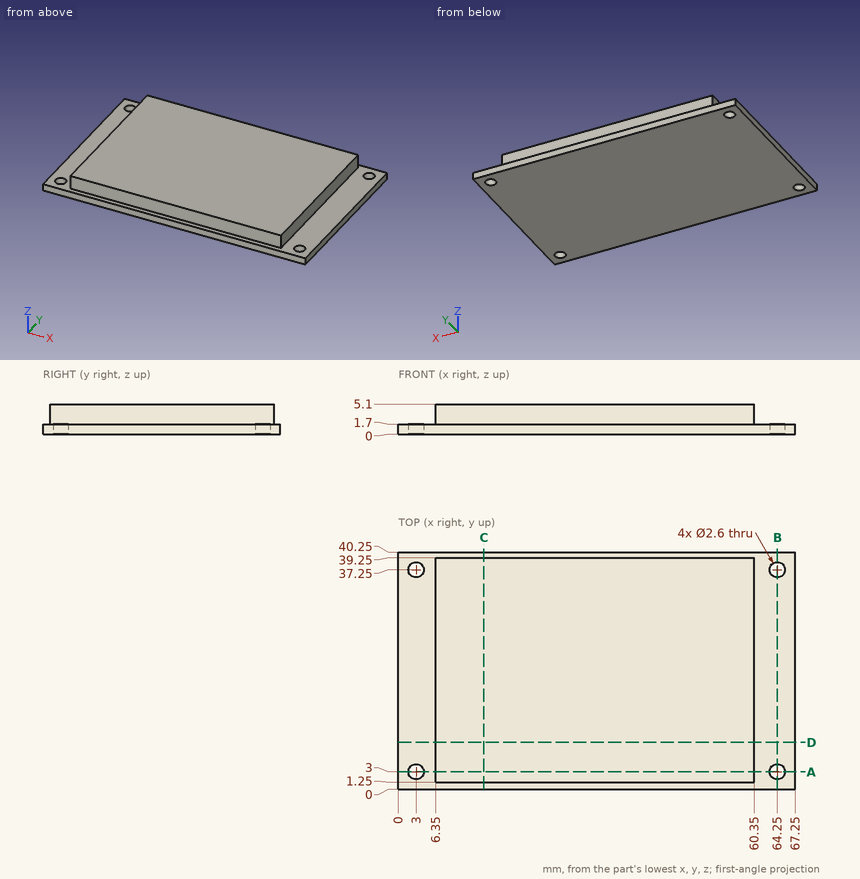
Job drawing, mm, ordinate dimensions from the low corner. One solid piece. Give positions to 0.01 mm unless a question says otherwise; leave off trailing zeros. Order: outer loops, then holes, each group sorted by start corner. A loop starts at its lowest first (then second) coordinate and runs counter-clockwise, first axis right, second up. Notation, with made-up numbers: M 81,5 L 114,5 A28 ccw 114,30 Z; hole C 7.5,88.5 d1. An arc over 180 degrees is marked long. Return JSON: item names as keys, results as strings.
Q1. Band-saw the part on D-D (y = 8). Give the cut face in (x, z).
Answer list:
{"outline": "M 0,0 L 67.25,0 L 67.25,1.7 L 60.35,1.7 L 60.35,5.1 L 6.35,5.1 L 6.35,1.7 L 0,1.7 Z"}
Q2. Flat gauge pins, fed straight in: pin 1 (1.6 mm diameter, centred on x = 64.25, y = 3, fed in from +Z); pin 2 (3.5 mm diameter, centred on x = 3, y = 3, fed in from +Z); pin 3 (3 mm diameter, centred on y = 15.5, z = 3.5, fed in from +X). Where does each tip first touch, or does it go through?
Answer list:
{"pin 1": "passes through", "pin 2": "stops at z = 1.7", "pin 3": "stops at x = 60.35"}
Q3. Wall check: probe 1 along Y at (x, z) = (3, 1.35); probe 2 along Y at (x, z) = (52, 2); probe 3 along X at (y, z) = (34.5, 2.6). Give the ranges that are in metal, low to high. Write a range as from..to.
Answer list:
{"probe 1": "y = 0..1.7, 4.3..35.95, 38.55..40.25", "probe 2": "y = 1.25..39.25", "probe 3": "x = 6.35..60.35"}
Q4. Band-saw the part on A-A (y = 3). Give the cut face in (x, z).
Answer list:
{"outline": "M 0,0 L 1.7,0 L 1.7,1.7 L 0,1.7 Z; M 4.3,0 L 62.95,0 L 62.95,1.7 L 60.35,1.7 L 60.35,5.1 L 6.35,5.1 L 6.35,1.7 L 4.3,1.7 Z; M 65.55,0 L 67.25,0 L 67.25,1.7 L 65.55,1.7 Z"}
Q5. Band-saw the part on C-C (x = 14.5). Give the cut face in (y, z).
Answer list:
{"outline": "M 0,0 L 40.25,0 L 40.25,1.7 L 39.25,1.7 L 39.25,5.1 L 1.25,5.1 L 1.25,1.7 L 0,1.7 Z"}
Q6. Band-saw the part on B-B (x = 64.25). Give the cut face in (y, z).
Answer list:
{"outline": "M 0,0 L 1.7,0 L 1.7,1.7 L 0,1.7 Z; M 4.3,0 L 35.95,0 L 35.95,1.7 L 4.3,1.7 Z; M 38.55,0 L 40.25,0 L 40.25,1.7 L 38.55,1.7 Z"}
